The figure shows three views and two pictorial views of one solid part (mm, origin at its lowest corner). Answer the questions. Coordinates: 2 decimals unless noted, no trailing zeros. Loops run counter-clockwise (first coordinate to the right, second up) from the corner with the lowest first, then second, coordinate; pieces in that order, holes last. Notation, with made-up numbers: M 74,-38 L 85,-38 A15 cw 85,-28 Z; hole C 88.25,43.5 d11. An arc over 180 degrees is marked long. Write each question's results on one line, items separated by ' | '.
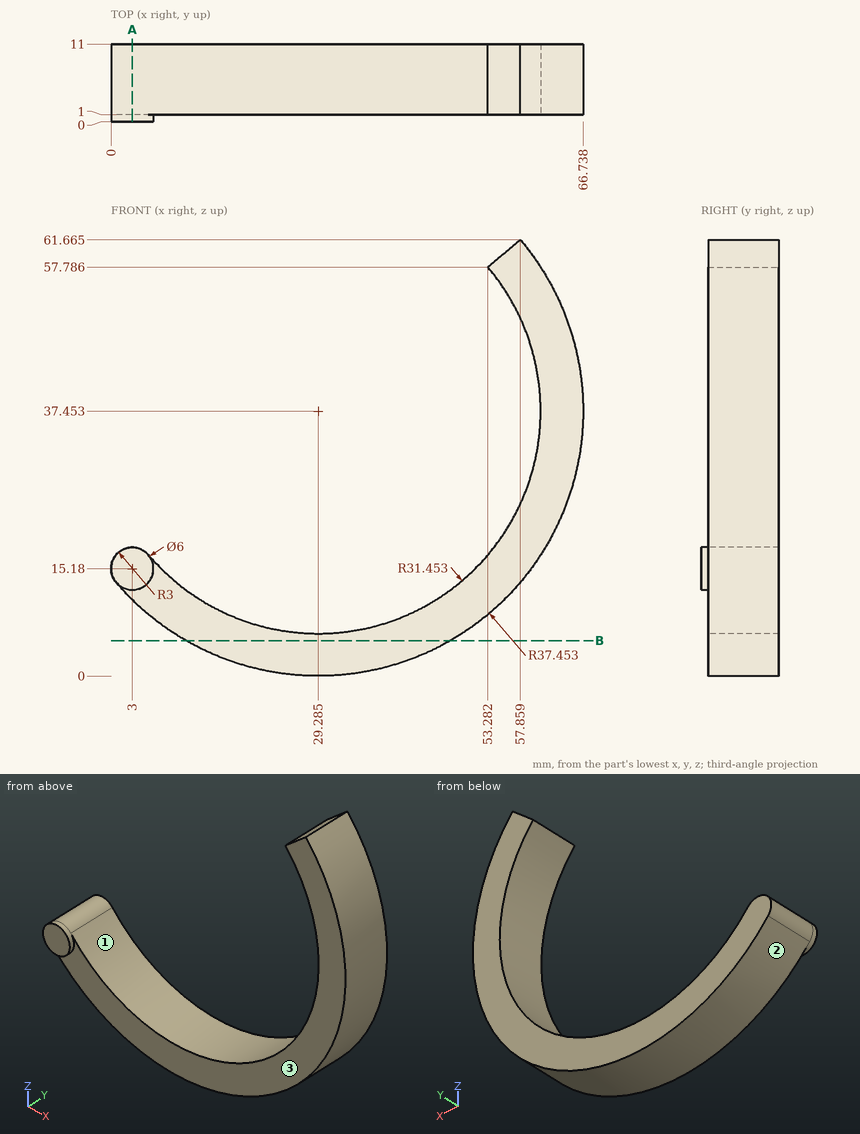
1) Straight lines are drawn through the part: probe 1 along X at (y, z) = (8.25, 15) (1 decimal); probe 2 along Y at (x, z) = (63, 34); probe 3 along Z at (x, y) = (28.5, 8). For each, find the intervals that lie inside material, in ascending order. Write a range as [from, to].
Check result:
probe 1: [0, 7.3], [51.3, 59.3] | probe 2: [1, 11] | probe 3: [0.01, 6.01]
2) Given pin 1 Ø5 at (x, y) = (12.5, 10) entering from -Z; pin 2 Ø10 at (x, z) = (56.5, 13.5) entering from -Y; pin 3 Ø3 at (y, z) = (3.5, 34) entering from +X, each flat-ended and moving along its own axis, determine where each tip first touches the part or whether it passes through.
Check result:
pin 1: z = 2.83 | pin 2: y = 1 | pin 3: x = 66.69
3) For a pull along X with two mould halves and no side action, classify the marked faces 1, 2 and 3 as released by +X, released by -X, zero draft, split by the parting line, or undercut.
Check result:
face 1: undercut | face 2: split by the parting line | face 3: zero draft
4) Find section B-B, the plane z = 5. Give the vertices of the cut face in (x, y).
Check result:
outline: M 10.59,1 L 47.98,1 L 47.98,11 L 10.59,11 Z
5) Find section A-A, the plane x = 3. Give the vertices of the cut face in (y, z).
Check result:
outline: M 0,12.18 L 1,12.18 L 1,10.77 L 11,10.77 L 11,18.18 L 0,18.18 Z
